The listing builds one solid part. Answer for the finished solid, in the listing's coordinates (mm). A direction names the side the tool comes from. Coordinates: 2 decimals unless noted, no trailing zeros. Loops run counter-clockwise (first coordinate to the right, second up) from the corner with the lowest first, then second, coordinate; pieces in that order, holes last. Notation, with made-up numbers: M 55.25,-30 L 91.25,-30 A3 cw 91.25,-26 Z; hole C -5,83 d5. An arc over 180 degrees is marked long. Return JSON: item names as keys, results as strings. Group by question number.
1. The mould has two halves that part along X. Classify faces 1 (the face through (-8.652, -0.783, -5.625)), 2 (the face through (1.588, -16, -12)), 3 (the face through (-17.135, -0.783, -20.518)), 4 (the face through (-13, -1.588, -13)): pulls with the +X half, pulls with the -X half, needs draft (parallel to the pull), parting line crosses it, or undercut.
2. Section C-C (x = -3.5) is taken. Write down the section's boundary in (y, z).
3. Section A-A (z = -6.35) is taken. Write down the section's boundary in (x, y).
4. Straight lines are drawn through the part: L1, parallel to Z at x = -6.35, y = -0.7; L2, parallel to Z at x = -12.75, y = -20.5. For each, find the intervals that lie inside material, in ascending order. Write a range as from..to.
5. Which of the six approach directions +Z, -Z, +X, -X, +Y, -Y give full straight-line access (tool end or side, diameter ignored) to faces 5 (the face through (0, -17, -13)), 6 (the face through (0.2, -32.068, -5.8))?
6. Section B-B (x = -19.05) is taken. Write down the section's boundary in (y, z).
7. Given P1, Ø1, axis at y = -10.5, z = -2.5, coming from the -X side; P2, Ø7.5, axis at y = -25.72, z = -12.7, coming from the +X side; P3, Ø4, axis at x = -19, y = -10, coming from the -Z side; P4, Ø7.5, axis at x = -16.5, z = -8, coming from the -Y side, each flat-ended and moving along its own axis, determine where each tip first touches the part or whether it passes through.
8. Section D-D (z = -1) is taken. Write down the section's boundary in (x, y), then the cut area to 3 significant figures.
Autodesk Inventor part; units mm, degrees
ref_plane "YZ Plane" through (0, 0, 0) normal (1, 0, 0) x (0, 1, 0)
ref_plane "XZ Plane" through (0, 0, 0) normal (0, 1, 0) x (-1, 0, 0)
ref_plane "XY Plane" through (0, 0, 0) normal (0, 0, 1) x (1, 0, 0)
sketch "Sketch1" plane through (0, 0, 0) normal (0, 1, 0) x (-1, 0, 0)
  line L0 (0, 0) -> (25.4, 0)
  line L1 (25.4, 0) -> (25.4, -25.4)
  line L2 (25.4, -25.4) -> (0, -25.4)
  line L3 (0, -25.4) -> (0, 0)
  line L4 (-1.5875, 1.5875) -> (26.9875, 1.5875)
  line L5 (26.9875, 1.5875) -> (26.9875, -26.9875)
  line L6 (26.9875, -26.9875) -> (-1.5875, -26.9875)
  line L7 (-1.5875, -26.9875) -> (-1.5875, 1.5875)
  circle A0 centre (19.05, -6.35) radius 2.413
  circle A1 centre (19.05, -19.05) radius 2.413
  circle A2 centre (6.35, -6.35) radius 2.413
  circle A3 centre (6.35, -19.05) radius 2.413
  dimension "d0" = 25.4
  dimension "d1" = 25.4
  dimension "d2" = 1.5875
  dimension "d3" = 6.35
  dimension "d4" = 6.35
  dimension "d5" = 4.826
  dimension "d8" = 12.7
  dimension "d11" = 12.7
extrude "Extrusion1" add sketch "Sketch1" against normal blind 1.5875 contours L0 L1 L2 L3 | L4 L5 L6 L7
extrude "Extrusion2" add sketch "Sketch1" against normal blind 32.0675 contours L4 L5 L6 L7
sketch "Sketch2" plane through (1.5875, 0, 1.5875) normal (1, 0, 0) x (0, 0, -1)
  line L0 (0, 0) -> (28.575, 0) construction
  line L1 (14.2875, 0) -> (14.2875, -32.0675) construction
  line L2 (26.9875, -32.0675) -> (1.5875, -32.0675) construction
  circle A0 centre (14.2875, -6.35) radius 2.413
  circle A1 centre (14.2875, -25.7175) radius 2.413
  point P0 (1.5875, 0)
  dimension "d18" = 4.826
  dimension "d19" = 4.826
  dimension "d20" = 6.35
  dimension "d21" = 6.35
extrude "Extrusion3" cut sketch "Sketch2" against normal blind 32.0675
sketch "Sketch3" plane through (-26.9875, 0, -26.9875) normal (-1, 0, 0) x (0, 0, 1)
  circle A0 centre (14.2875, -25.7175) radius 2.413
  circle A1 centre (14.2875, -6.35) radius 2.413
  line L0 (0, 0) -> (28.575, 0)
  line L1 (0, 0) -> (0, -32.0675)
  line L2 (28.575, -32.0675) -> (0, -32.0675)
  line L3 (28.575, 0) -> (28.575, -32.0675)
  point P0 (26.9875, 0)
sketch "Sketch4" plane through (1.5875, 0, -26.9875) normal (0, 0, -1) x (-1, 0, 0)
  line L0 (0, 0) -> (28.575, 0)
  line L1 (0, 0) -> (0, -32.0675)
  line L2 (28.575, -32.0675) -> (0, -32.0675)
  line L3 (28.575, 0) -> (28.575, -32.0675)
  point P0 (1.5875, 0)
extrude "Extrusion4" cut sketch "Sketch3" against normal blind 1.5875
extrude "Extrusion5" cut sketch "Sketch4" against normal blind 1.5875
equation "\"d18\" = d19"
equation "\"d21\" = d20"
properties part number "FlipperTensionerBlock2Tool"
Worked out:
{
 "1": {"face 1": "undercut", "face 2": "pulls with the +X half", "face 3": "undercut", "face 4": "needs draft"},
 "2": {"outline": "M -32.07,0 L -1.59,0 L -1.59,-25.4 L 0,-25.4 L 0,1.59 L -32.07,1.59 Z"},
 "3": {"outline": "M -25.4,-1.59 L -21.46,-1.59 L -21.46,0 L -25.4,0 Z; M -16.64,-1.59 L -8.76,-1.59 L -8.76,0 L -16.64,0 Z; M -3.94,-1.59 L 0,-1.59 L 0,-32.07 L 1.59,-32.07 L 1.59,0 L -3.94,0 Z"},
 "4": {"L1": "-25.4..-21.46, -16.64..-8.76, -3.94..1.59", "L2": "0..1.59"},
 "5": {"face 5": "-Z, -X, -Y", "face 6": "+Z, -Z, +X, -X, -Y"},
 "6": {"outline": "M -32.07,0 L -1.59,0 L -1.59,-3.94 L 0,-3.94 L 0,1.59 L -32.07,1.59 Z; M -1.59,-25.4 L 0,-25.4 L 0,-21.46 L -1.59,-21.46 Z; M -1.59,-16.64 L 0,-16.64 L 0,-8.76 L -1.59,-8.76 Z"},
 "7": {"P1": "x = 0", "P2": "x = 1.59", "P3": "z = 0", "P4": "y = -1.59"},
 "8": {"outline": "M -25.4,-1.59 L 0,-1.59 L 0,-32.07 L 1.59,-32.07 L 1.59,0 L -25.4,0 Z", "area": "91.2 mm^2"}
}
